Design review of the part built by this model. Coordinates are the model's own, in mm. Coordinates: 2 decimals unless noted, no trailing zeros. Order: outer loops, then holes, each group sorted by start corner. A loop starts at its lowest first (then second) coordinate and runs counter-clockwise, first axis right, second up. Notation, with made-up numbers: (86.25, 57.5) -> (100.25, 57.5) arc R15 ccw to (100.25, 63.5) -> close; hole circle Ø8 at (-31, -5). An arc over 180 degrees is marked (long way). Use a Markdown table: item, result. Add a question column.
Q1. Add section C-C (x = 222.5). State the section outline as (y, z) points.
Q2. Add section A-A (z = -0.8). State the section outline as (x, y) points, then the cut area to 3 significant figures.
Q3. Insertion check: pin 1 (5 mm diameter, centred on x = 300, y = 116.08, fed in from -Z). The pin has a flat end and moves straight along its axis. Give the tip position at first contact, or say it passes through.
Q4. Add section B-B (y = 179.5). State the section outline as (x, z) points, then the cut area to 3 significant figures.
Q5. Wall thickness on probe 1 along Y at (x, z) = (0, -0.65); probe 2 along X at (y, z) = (489, -0.7); probe 3 along Y at (x, z) = (-300, -0.5): over which ranges is each line inside the solid? List them lowest first.
from build123d import *

# Parameters (mm, degrees)
SM_BASE_FLANGE_1_DEPTH = 1
SKETCH_2_R             = 3
CUT_EXTRUDE_1_DEPTH    = 815.794452608


# Sheet-metal steps are written as plain solids
with BuildPart() as part:
    # Sketch 1 → Базовая кромка1 (new body)
    with BuildSketch(Plane.XY):
        with BuildLine():
            Line((-306.267856622, 0), (306.267856622, 0))
            ThreePointArc((306.267856622, 0), (0, 700), (-306.267856622, 0))
        make_face()
    extrude(amount=-SM_BASE_FLANGE_1_DEPTH)

    # Эскиз2 → Вырез-Вытянуть1 (cut, through all)
    with BuildSketch(Plane.XY):
        with Locations((-300, 116.083573562)):
            Circle(SKETCH_2_R)
        with Locations((300, 116.083573562)):
            Circle(SKETCH_2_R)
        with Locations((0, 695)):
            Circle(SKETCH_2_R)
        with Locations((356.802466359, 489)):
            Circle(SKETCH_2_R)
        with Locations((-356.802466359, 489)):
            Circle(SKETCH_2_R)
    extrude(amount=-CUT_EXTRUDE_1_DEPTH, mode=Mode.SUBTRACT)


solid = part.part
Established:
| question | item | result |
|---|---|---|
| 1 | outline | (0, -1) -> (635.68, -1) -> (635.68, 0) -> (0, 0) -> close |
| 2 | outline | (-306.27, 0) -> (306.27, 0) arc R417 ccw (long way) to start; hole circle Ø6 at (-356.8, 489); hole circle Ø6 at (-300, 116.08); hole circle Ø6 at (0, 695); hole circle Ø6 at (300, 116.08); hole circle Ø6 at (356.8, 489) |
| 2 | area | 489,000 mm^2 |
| 3 | pin 1 | through |
| 4 | outline | (-403.95, -1) -> (403.95, -1) -> (403.95, 0) -> (-403.95, 0) -> close |
| 4 | area | 808 mm^2 |
| 5 | probe 1 | 0 to 692, 698 to 700 |
| 5 | probe 2 | -362.56 to -359.8, -353.8 to 353.8, 359.8 to 362.56 |
| 5 | probe 3 | 0 to 113.08, 119.08 to 572.64 |
